Part model, mm, in its own coordinate system. Face numbers are marked on the shaded views. A direction names the side the tool comes from. Round coordinates to 2 decimals unless told otherwise and drop trailing zeros. Write each loop counter-clockwise with the first axis right and the second up, starting at its lowest first coordinate (ties: lowest second). Pieces come first, ordered by that corner, then holes.
1) Pull direction X, two halves, no side cores. Call the marked faces 5, 6 and 7: +X half, -X half, draft (parallel to the pull), parting line (faces both ways), or undercut.
2) Flat gauge pins, fed straight in: pin 1 (12 mm diameter, centred on x = -2, z = -8.5, fed in from -Y); pin 2 (6 mm diameter, centred on x = 9, y = -24.5, fed in from -Z); pin 3 (8.5 mm diameter, centred on x = -13.45, y = -36.58, fed in from +Z); pin 4 (5.5 mm diameter, centred on x = -11.5, y = -39, fed in from -Z). Where does each tip first touch, or does it go through?
3) Drill centre lines: L1, parallel to Z at x = 21, y = -34.5; L2, parallel to Z at x = -14, y = -66; L3, parallel to X at y = -15, z = -2.5. Where is each one in solid material? Low to high.
4) Saw through at C-C on z = -29. Write the cut outline in (x, y).
5) Saw through at A-A on x = -13.5. Write the cut outline in (y, z), and give its area (3 significant figures).
6) Saw through at D-D on x = 13.5. Write the cut outline in (y, z), and give its area (3 significant figures).
7) Saw through at B-B on y = -45. Write the cut outline in (x, z) (3 decimals).
8) Which spindle directions (+Z, -Z, +X, -X, +Y, -Y) get a long thin tool onto all of the face, cutting with end or side? Do the marked faces 1, 2, 3 and 4. Say none if no direction does.
```python
from build123d import *

# Parameters (mm, degrees)
F1_DEPTH = 73.152
F3_D     = 6.5278
F5_DEPTH = 47.626
F6_R     = 3.175


with BuildPart() as f1:
    # F0 (on Front) → F1 (new body)
    with BuildSketch(Plane.XZ):
        Polygon((32.5217237333, 11.9879317781), (32.5217237333, 15.1629317781), (-1.7682762667, 15.1629317781), (-1.7682762667, -26.9058182219), (-27.6762762667, -26.9058182219), (-27.6762762667, -32.4620682219), (-22.6597762667, -32.4620682219), (-22.6597762667, -30.0808182219), (-3.6097762667, -30.0808182219), (-3.6097762667, -32.4620682219), (1.4067237333, -32.4620682219), (1.4067237333, 11.9879317781), (30.1404737333, 11.9879317781), (30.1404737333, 8.8129317781), (32.5217237333, 8.8129317781), align=None)
    extrude(amount=F1_DEPTH)

    # F3 (through all)
    with Locations(Plane(origin=(0, 0, -30.0808182219), x_dir=(1, 0, 0), z_dir=(0, 0, -1))):
        with Locations((-13.4522762667, 13.716), (-13.4522762667, 36.576), (-13.4522762667, 59.436)):
            Hole(F3_D / 2)

    # F4 (on face) → F5 (cut, through all)
    with BuildSketch(Plane.XY.offset(15.1629317781)):
        with BuildLine():
            ThreePointArc((20.3297237333, -27.3588467389), (15.5037237333, -22.5328467389), (10.6777237333, -27.3588467389))
            Line((10.6777237333, -27.3588467389), (10.6777237333, -43.1068467389))
            ThreePointArc((10.6777237333, -43.1068467389), (15.5037237333, -47.9328467389), (20.3297237333, -43.1068467389))
            Line((20.3297237333, -43.1068467389), (20.3297237333, -27.3588467389))
        make_face()
    extrude(amount=-F5_DEPTH, mode=Mode.SUBTRACT)

    # F6
    f6_edges = [f1.edges().sort_by_distance(p)[0] for p in [
        (-1.768276, -36.576, -26.905818),
        (1.406724, -36.576, 11.987932),
        (-27.676276, -36.576, -26.905818),
    ]]
    fillet(f6_edges, radius=F6_R)


solid = f1.part
```
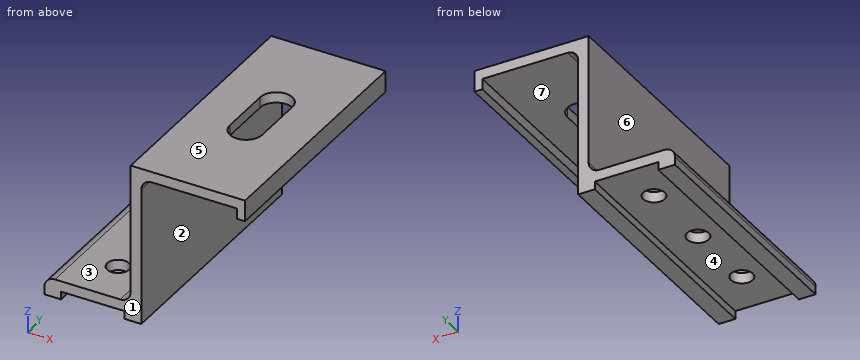
Completed:
1. face 5: draft
1. face 6: -X half
1. face 7: undercut
2. pin 1: stops at y = -73.15
2. pin 2: stops at z = 11.99
2. pin 3: stops at z = -26.91
2. pin 4: stops at z = -30.08
3. L1: z = 11.99 to 15.16
3. L2: z = -30.08 to -26.91
3. L3: x = -1.77 to 1.41
4. outline: (-27.49, -73.15) - (1.41, -73.15) - (1.41, 0) - (-27.49, 0) - close; hole circle Ø6.53 at (-13.45, -59.44); hole circle Ø6.53 at (-13.45, -36.58); hole circle Ø6.53 at (-13.45, -13.72)
5. outline: (-73.15, -30.08) - (-62.7, -30.08) - (-62.7, -26.91) - (-73.15, -26.91) - close; (-56.17, -30.08) - (-39.84, -30.08) - (-39.84, -26.91) - (-56.17, -26.91) - close; (-33.31, -30.08) - (-16.98, -30.08) - (-16.98, -26.91) - (-33.31, -26.91) - close; (-10.45, -30.08) - (0, -30.08) - (0, -26.91) - (-10.45, -26.91) - close
5. area: 170 mm2
6. outline: (-73.15, 11.99) - (-47.5, 11.99) - (-47.5, 15.16) - (-73.15, 15.16) - close; (-22.97, 11.99) - (0, 11.99) - (0, 15.16) - (-22.97, 15.16) - close
6. area: 154 mm2
7. outline: (-27.676, -32.462) - (-22.66, -32.462) - (-22.66, -30.081) - (-3.61, -30.081) - (-3.61, -32.462) - (1.407, -32.462) - (1.407, 8.813) arc R3.175 cw to (4.582, 11.988) - (11.065, 11.988) - (11.065, 15.163) - (-1.768, 15.163) - (-1.768, -23.731) arc R3.175 cw to (-4.943, -26.906) - (-24.501, -26.906) arc R3.175 ccw to (-27.676, -30.081) - close; (19.943, 11.988) - (30.14, 11.988) - (30.14, 8.813) - (32.522, 8.813) - (32.522, 15.163) - (19.943, 15.163) - close
8. face 1: +Z, -Z, +X, -X, -Y
8. face 2: -Z, +X, +Y, -Y
8. face 3: +Z, -X, +Y, -Y
8. face 4: -Z, +Y, -Y
